Model file for the job. Use its own axes, mm. Face numbers are marked on the shaded views. Coordinates: 2 decimals unless noted, no trailing zeros. Loops run counter-clockwise (first coordinate to the right, second up) from the corner with the lowest first, then second, coordinate; pieces in that order, holes last. Notation, with made-up numbers: (36, 85.25) - (77, 85.25) arc R21 cw to (77, 120.25) - close; hole circle Ø3 at (-36, -20.75). An arc over 180 degrees is marked (long way). Write each question's results on one line, items separated by ' | '. Start each with the question number.
```python
from build123d import *

# Parameters (mm, degrees)
F0_R     = 10
F0_R_2   = 11.5
F1_DEPTH = 13


with BuildPart() as f1:
    # F0 (on Top) → F1 (new body)
    with BuildSketch(Plane.XY):
        with BuildLine():
            ThreePointArc((12.111219, 26.367962), (16.096526, 32.133281), (17.5, 39))
            ThreePointArc((17.5, 39), (-5.334249, 55.667207), (-14.24809, 28.839196))
            ThreePointArc((-14.24809, 28.839196), (-1.633494, 21.576404), (12.111219, 26.367962))
        make_face()
        with Locations((0, 39)):
            Circle(F0_R, mode=Mode.SUBTRACT)
        with BuildLine():
            ThreePointArc((11.283926, 9.882966), (-1.294732, 14.944018), (-12.815525, 7.795019))
            ThreePointArc((-12.815525, 7.795019), (-14.959668, -1.099247), (-11.53846, -9.584568))
            ThreePointArc((-11.53846, -9.584568), (0.525844, -14.99078), (12.181685, -8.752517))
            ThreePointArc((12.181685, -8.752517), (14.278047, -4.597539), (15, 0))
            ThreePointArc((15, 0), (14.040279, 5.279257), (11.283926, 9.882966))
        make_face()
        Circle(F0_R_2, mode=Mode.SUBTRACT)
        with BuildLine():
            ThreePointArc((12.111219, 26.367962), (-1.633494, 21.576404), (-14.24809, 28.839196))
            ThreePointArc((-14.24809, 28.839196), (-10.554394, 18.519793), (-12.815525, 7.795019))
            ThreePointArc((-12.815525, 7.795019), (-1.294732, 14.944018), (11.283926, 9.882966))
            ThreePointArc((11.283926, 9.882966), (9.280567, 18.246761), (12.111219, 26.367962))
        make_face()
        with BuildLine():
            ThreePointArc((12.181685, -8.752517), (0.525844, -14.99078), (-11.53846, -9.584568))
            ThreePointArc((-11.53846, -9.584568), (-9.368827, -17.888551), (-11.835438, -26.109212))
            ThreePointArc((-11.835438, -26.109212), (-0.036151, -21.500037), (11.782078, -26.060424))
            ThreePointArc((11.782078, -26.060424), (9.453579, -17.348097), (12.181685, -8.752517))
        make_face()
        with BuildLine():
            ThreePointArc((11.782078, -26.060424), (-0.036151, -21.500037), (-11.835438, -26.109212))
            ThreePointArc((-11.835438, -26.109212), (-7.040236, -55.021394), (17.5, -39))
            ThreePointArc((17.5, -39), (16.006817, -31.926683), (11.782078, -26.060424))
        make_face()
        with Locations((0, -39)):
            Circle(F0_R, mode=Mode.SUBTRACT)
    extrude(amount=F1_DEPTH)


solid = f1.part
```
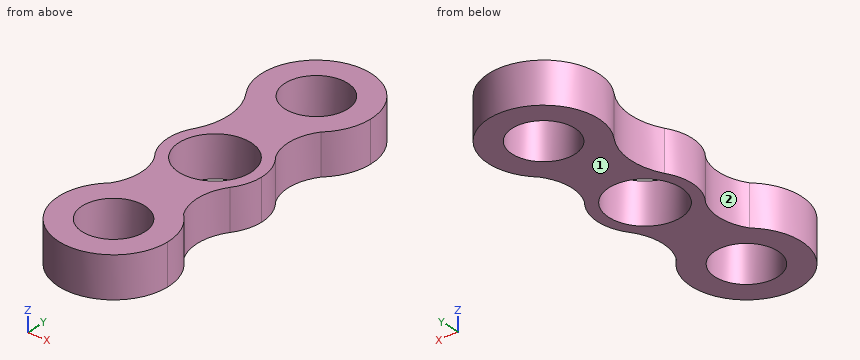
Q1. Cut at B-B (y = -45.5). List the corners of the cut face in (x, z).
Q2. Mould opens along Y. For the marked faces 1 and 2 say: +Y half, -Y half, draft (parallel to the pull), parting line (faces both ways), or undercut.
Q3. Cut at C-C (z = 8.5). List the corners of the cut face in (x, y).
Q4. Cut at D-D (y = 40). List the corners of the cut face in (x, z), and give its area (3 significant figures).
Q5. Pin check, flat tips, straight feed: pin 1 (4 mm diameter, centred on x = 8.5, z = 4.5, fed in from -Y); pin 2 (3 mm diameter, centred on x = 10, z = 10.5, fed in from +Y); pin 3 (1 mm diameter, centred on y = 8.5, z = 2.5, fed in from +X). Stop position of each tip, or through.
Q6. Drill centre lines: L1, parallel to Y at x = 0, z = 10.25; L2, parallel to Y at x = 6, z = 1.5; L3, parallel to X at y = 9, z = 5.25. Where is each one in solid material? Low to high. Write a range as from..to.
Q7. Cut at A-A (x = 0). List the corners of the cut face in (y, z), and give its area (3 significant figures).
Check result:
1) outline: (-16.25, 0) - (-7.6, 0) - (-7.6, 13) - (-16.25, 13) - close; (7.6, 0) - (16.25, 0) - (16.25, 13) - (7.6, 13) - close
2) face 1: draft | face 2: undercut
3) outline: (-14.25, 28.84) arc R20.13 cw to (-12.82, 7.8) arc R15 ccw to (-11.54, -9.58) arc R15.89 cw to (-11.84, -26.11) arc R17.5 ccw (long way) to (17.5, -39) arc R17.5 ccw to (11.78, -26.06) arc R16.08 cw to (12.18, -8.75) arc R15 ccw to (15, 0) arc R15 ccw to (11.28, 9.88) arc R15.28 cw to (12.11, 26.37) arc R17.5 ccw to (17.5, 39) arc R17.5 ccw (long way) to start; hole circle Ø23 at (0, 0); hole circle Ø20 at (0, -39); hole circle Ø20 at (0, 39)
4) outline: (-17.47, 0) - (-9.95, 0) - (-9.95, 13) - (-17.47, 13) - close; (9.95, 0) - (17.47, 0) - (17.47, 13) - (9.95, 13) - close | area: 196 mm²
5) pin 1: y = -55.25 | pin 2: y = 54.3 | pin 3: x = 12.69
6) L1: -56.5..-49, -29..-11.5, 11.5..29, 49..56.5 | L2: -55.44..-47, -31..-9.81, 9.81..31, 47..55.44 | L3: -12.23..-7.16, 7.16..12
7) outline: (-56.5, 0) - (-49, 0) - (-49, 13) - (-56.5, 13) - close; (-29, 0) - (-11.5, 0) - (-11.5, 13) - (-29, 13) - close; (11.5, 0) - (29, 0) - (29, 13) - (11.5, 13) - close; (49, 0) - (56.5, 0) - (56.5, 13) - (49, 13) - close | area: 650 mm²
